```python
from build123d import *

# Parameters (mm, degrees)
BOSS_EXTRUDE1_DEPTH = 6.35
CUT_EXTRUDE1_REACH  = 15.395
SKETCH2_R           = 1.651
CUT_EXTRUDE2_REACH  = 15.49
SKETCH3_R           = 1.4224


with BuildPart() as part:
    # Sketch1 → Boss-Extrude1 (new body)
    with BuildSketch(Plane(origin=(0, 0, 0), x_dir=(0, 0, -1), z_dir=(1, 0, 0))):
        Polygon((0, 0), (0, 8.7122), (-1.5748, 8.7122), (-1.5748, 1.5748), (-9.525, 1.5748), (-9.525, 0), align=None)
    extrude(amount=-BOSS_EXTRUDE1_DEPTH)

    # Sketch2 → Cut-Extrude1 (cut, up to next)
    with BuildSketch(Plane.XY.offset(1.5748), mode=Mode.PRIVATE) as cut_extrude1_sk1:
        with Locations((-3.175, 5.1562)):
            Circle(SKETCH2_R)
    cut_extrude1_tool1 = extrude(cut_extrude1_sk1.sketch, amount=-CUT_EXTRUDE1_REACH, mode=Mode.PRIVATE) & part.part
    add(cut_extrude1_tool1.solids().sort_by_distance((-3.175, 5.1562, 1.5748))[0], mode=Mode.SUBTRACT)

    # Sketch3 → Cut-Extrude2 (cut, up to next)
    with BuildSketch(Plane(origin=(0, 1.5748, 0), x_dir=(1, 0, 0), z_dir=(0, 1, 0)), mode=Mode.PRIVATE) as cut_extrude2_sk1:
        with Locations(Location((-3.175, -6.35, 0), (0, 0, 270))):
            Circle(SKETCH3_R)
    cut_extrude2_tool1 = extrude(cut_extrude2_sk1.sketch, amount=-CUT_EXTRUDE2_REACH, mode=Mode.PRIVATE) & part.part
    add(cut_extrude2_tool1.solids().sort_by_distance((-3.175, 1.5748, 6.35))[0], mode=Mode.SUBTRACT)


solid = part.part
```
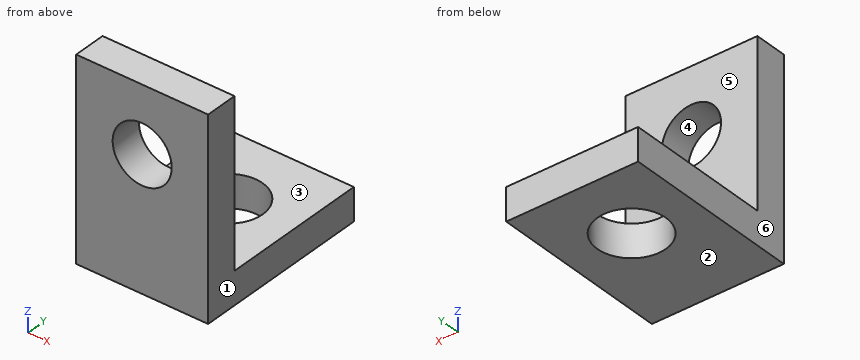
Check sheet for the modelled part. Datum: model origin and axes. Units: mm. Face numbers are marked on the shaded views. A direction names the side the tool comes from. Round coordinates to 2 decimals unless told otherwise and drop trailing zeros. Order: outer loops, then holes, each group sorted by start corner. A loop starts at its lowest first (then second) coordinate and runs counter-clockwise, first axis right, second up.
1) Section check B-B (x = -4.25). Record the boundary of the cut face in (y, z) (3 decimals).
2) Tool access check on the marked faces 5 and 6. Record the directions out of +Z, -Z, +X, -X, +Y, -Y that give a thin tool (end or side, any length) a straight path to the whole face; none if there is none.
3) Section check A-A (z = 6.25). Record the boundary of the cut face in (x, y), and give its area (3 significant figures).
4) Scan lines: line 1 (X direction, y = 1.2, z = 6.35); line 2 (Y direction, x = -5.25, z = 3.25). Record each from-to range of solid material in increasing order.
5) Section check C-C (y = 5). Record the boundary of the cut face in (x, z), and give its area (3 significant figures).
6) Mould release check, pull along Z, two halves, no side actions. Record for the marked faces 1, 2, 3 and 4: +Z half, -Z half, draft (parallel to the pull), parting line (faces both ways), or undercut.
7) Section check D-D (z = 1.75). Record the boundary of the cut face in (x, y).
Result:
1. outline: (0, 0) - (3.903, 0) - (3.903, 1.575) - (1.575, 1.575) - (1.575, 5.419) - (0, 5.419) - close; (0, 7.281) - (1.575, 7.281) - (1.575, 9.525) - (0, 9.525) - close; (6.409, 0) - (8.712, 0) - (8.712, 1.575) - (6.409, 1.575) - close
2. face 5: +Z, +X, -X, +Y
2. face 6: +Z, -Z, -X, +Y, -Y
3. outline: (-6.35, 0) - (-4.59, 0) - (-4.59, 1.57) - (-6.35, 1.57) - close; (-1.76, 0) - (0, 0) - (0, 1.57) - (-1.76, 1.57) - close
3. area: 5.53 mm2
4. line 1: x = -6.35 to -4.6, -1.75 to 0
4. line 2: y = 0 to 1.57
5. outline: (-6.35, 0) - (-4.82, 0) - (-4.82, 1.57) - (-6.35, 1.57) - close; (-1.53, 0) - (0, 0) - (0, 1.57) - (-1.53, 1.57) - close
5. area: 4.82 mm2
6. face 1: draft
6. face 2: -Z half
6. face 3: +Z half
6. face 4: undercut
7. outline: (-6.35, 0) - (0, 0) - (0, 1.57) - (-6.35, 1.57) - close
